Could you check a few things on this model? Use its own coordinates, in mm. A direction names the side the tool comes from. Give positions to 0.01 mm unless a question says otherwise; leave off trailing zeros. Loops run counter-clockwise (first coordinate to the right, second up) from the corner with the lowest first, then second, coordinate; pieces in that order, holes last. Notation, with made-up numbers: M -11.75,22 L 23.25,22 A34 ccw 23.25,55 Z; hole C -6,61.25 d11. An arc over 180 degrees is marked long. Use a Markdown table: item, result. Add a question column.
1) Suppose I cut it at B-B on x = 40.5. List the corners of the cut face in (y, z) for me.
2) Will these pins go through, and if not, where does the flat tip stop? pin 1 Ø4 at (x, z) = (105.5, 3.5) entering from -Y; pin 2 Ø5.5 at (x, y) = (18.2, 54.31) entering from +Z; pin 3 Ø2 at (x, z) = (191, 12.5) entering from +Y.
3) Suppose I cut it at A-A on y = 44. List the corners of the cut face in (x, z) for me, and give its area (3 significant figures).
4) We'd pull the mould along X, two halves only. Please class faces 1 (the cylindrical face through (20.89, 57.91, 12.29)), 2 (the cylindrical face through (-2.896, 24.969, 7.395)), 3 (the flat face through (217.772, 56.913, 7.395)): +X half, -X half, draft (parallel to the pull), parting line (faces both ways), or undercut.
5) If I drill on line 1 along Y through (x, z) = (75, 10.75); line 2 along X through (y, z) = (92.5, 13); line 3 along Y through (x, z) = (119, 9.5), over which ranges is the centre line in solid material (lowest first)? Write a range as [from, to].
6) Which directions (+Z, -Z, +X, -X, +Y, -Y) give clear straight access to the entire face, cutting with the end or side of a thin tool? Please do faces 4 (the cylindrical face through (229.443, 8.896, 7.395)), 5 (the cylindrical face through (172.725, 98.745, 7.395)), 6 (the flat face through (61, 88, 6.5)), 7 (the cylindrical face through (57.199, 98.723, 7.395)), 8 (the flat face through (169, 88, 8.5)).
```python
from build123d import *

# Parameters (mm, degrees)
EXTRUDE_7_DEPTH     = 15
CUT_EXTRUDE_1_DEPTH = 257.870857521
RIB_4_REACH         = 258.542
SKETCH_7_WALL_W     = 532.538559092
SKETCH_7_WALL_H     = 2
RIB_5_REACH         = 258.542
SKETCH_8_WALL_W     = 532.538559092
SKETCH_8_WALL_H     = 2
CUT_EXTRUDE_2_DEPTH = 257.870857521
CUT_EXTRUDE_3_DEPTH = 10
CUT_EXTRUDE_4_DEPTH = 257.870857521
EXTRUDE_8_DEPTH     = 2


with BuildPart() as part:
    # 草图3 → 凸台-拉伸7 (new body)
    with BuildSketch(Plane.XY):
        with BuildLine():
            Line((226.107883645, 4.564084021), (228.1313581, 6.587558476))
            ThreePointArc((228.1313581, 6.587558476), (229.452157682, 8.933123872), (229.365360937, 11.623598716))
            ThreePointArc((229.365360937, 11.623598716), (202.204022959, 54.721265071), (157.336152658, 78.846383531))
            ThreePointArc((157.336152658, 78.846383531), (156.176241581, 79.053674225), (155, 79.123092382))
            Line((155, 79.123092382), (75, 79.123092382))
            ThreePointArc((75, 79.123092382), (73.823758419, 79.053674225), (72.663847342, 78.846383531))
            ThreePointArc((72.663847342, 78.846383531), (27.795977041, 54.721265071), (0.634639063, 11.623598716))
            ThreePointArc((0.634639063, 11.623598716), (0.547842318, 8.933123872), (1.8686419, 6.587558476))
            Line((1.8686419, 6.587558476), (3.892116355, 4.564084021))
            ThreePointArc((3.892116355, 4.564084021), (4.038087075, 4.232340324), (3.921585186, 3.889136825))
            Line((3.921585186, 3.889136825), (3.278797577, 3.123092382))
            ThreePointArc((3.278797577, 3.123092382), (2.939119693, 2.946368462), (2.574022538, 3.0617655))
            ThreePointArc((2.574022538, 3.0617655), (-3.997102919, -0.152211219), (2.799416849, -2.857142857))
            ThreePointArc((2.799416849, -2.857142857), (4.567091757, -2.875182235), (4.549052379, -4.642857143))
            ThreePointArc((4.549052379, -4.642857143), (-2.777041025, -5.876907618), (-6.475265538, 0.566512328))
            Line((-6.475265538, 0.566512328), (-5.60370811, 10.528459309))
            ThreePointArc((-5.60370811, 10.528459309), (-2.837136411, 25.169145871), (2.769030559, 38.974018703))
            Line((2.769030559, 38.974018703), (21.426225279, 74.356346003))
            ThreePointArc((21.426225279, 74.356346003), (23.699524873, 77.563248735), (26.727922901, 80.069425417))
            Line((26.727922901, 80.069425417), (54.688883256, 97.596110672))
            ThreePointArc((54.688883256, 97.596110672), (57.236866172, 98.733768292), (60, 99.123092382))
            Line((60, 99.123092382), (170, 99.123092382))
            ThreePointArc((170, 99.123092382), (172.763133828, 98.733768292), (175.311116744, 97.596110672))
            Line((175.311116744, 97.596110672), (203.272077099, 80.069425417))
            ThreePointArc((203.272077099, 80.069425417), (206.300475127, 77.563248735), (208.573774721, 74.356346003))
            Line((208.573774721, 74.356346003), (227.230969441, 38.974018703))
            ThreePointArc((227.230969441, 38.974018703), (232.837136411, 25.169145871), (235.60370811, 10.528459309))
            Line((235.60370811, 10.528459309), (236.475265538, 0.566512328))
            ThreePointArc((236.475265538, 0.566512328), (232.777041025, -5.876907618), (225.450947621, -4.642857143))
            ThreePointArc((225.450947621, -4.642857143), (225.432908243, -2.875182235), (227.200583151, -2.857142857))
            ThreePointArc((227.200583151, -2.857142857), (233.997102919, -0.152211219), (227.425977462, 3.0617655))
            ThreePointArc((227.425977462, 3.0617655), (227.060880307, 2.946368462), (226.721202423, 3.123092382))
            Line((226.721202423, 3.123092382), (226.078414814, 3.889136825))
            ThreePointArc((226.078414814, 3.889136825), (225.961912925, 4.232340324), (226.107883645, 4.564084021))
        make_face()
        with BuildLine():
            Line((155, 79.123092382), (151.5, 79.123092382))
            ThreePointArc((151.5, 79.123092382), (151.75, 79.056105084), (151.933012702, 78.873092382))
            Line((151.933012702, 78.873092382), (153.208862747, 76.663255282))
            ThreePointArc((153.208862747, 76.663255282), (153.460925165, 76.447146931), (153.792778177, 76.436570515))
            ThreePointArc((153.792778177, 76.436570515), (158.62462258, 70.93131487), (151.301621364, 71.099282859))
            ThreePointArc((151.301621364, 71.099282859), (149.669687564, 71.778835706), (148.990134717, 70.146901906))
            ThreePointArc((148.990134717, 70.146901906), (155.784690615, 66.170630787), (161.428180194, 71.659505648))
            ThreePointArc((161.428180194, 71.659505648), (163.815160833, 75.214538736), (168.0781083, 75.6185384))
            ThreePointArc((168.0781083, 75.6185384), (162.752422297, 77.383187743), (157.336152658, 78.846383531))
            ThreePointArc((157.336152658, 78.846383531), (156.176241581, 79.053674225), (155, 79.123092382))
        make_face()
        with BuildLine():
            ThreePointArc((72.663847342, 78.846383531), (67.247577703, 77.383187743), (61.9218917, 75.6185384))
            ThreePointArc((61.9218917, 75.6185384), (66.184839167, 75.214538736), (68.571819806, 71.659505648))
            ThreePointArc((68.571819806, 71.659505648), (74.215309385, 66.170630787), (81.009865283, 70.146901906))
            ThreePointArc((81.009865283, 70.146901906), (80.330312436, 71.778835706), (78.698378636, 71.099282859))
            ThreePointArc((78.698378636, 71.099282859), (71.37537742, 70.93131487), (76.207221823, 76.436570515))
            ThreePointArc((76.207221823, 76.436570515), (76.539074835, 76.447146931), (76.791137253, 76.663255282))
            Line((76.791137253, 76.663255282), (78.066987298, 78.873092382))
            ThreePointArc((78.066987298, 78.873092382), (78.25, 79.056105084), (78.5, 79.123092382))
            Line((78.5, 79.123092382), (75, 79.123092382))
            ThreePointArc((75, 79.123092382), (73.823758419, 79.053674225), (72.663847342, 78.846383531))
        make_face()
    extrude(amount=EXTRUDE_7_DEPTH)

    # 草图6 → 切除-拉伸1 (cut, through all)
    with BuildSketch(Plane.XY.offset(15)):
        with BuildLine():
            ThreePointArc((58.67439973, 95.652604272), (57.292832816, 95.457942227), (56.018841358, 94.889113416))
            Line((56.018841358, 94.889113416), (51.236866172, 91.891642195))
            Line((51.236866172, 91.891642195), (51.236866172, 74.437432673))
            ThreePointArc((51.236866172, 74.437432673), (60.685741856, 78.429836873), (70.484678821, 81.463214092))
            ThreePointArc((70.484678821, 81.463214092), (71.026743583, 81.818757299), (71.236866172, 82.432022066))
            Line((71.236866172, 82.432022066), (71.236866172, 94.652604272))
            ThreePointArc((71.236866172, 94.652604272), (70.943972953, 95.359711053), (70.236866172, 95.652604272))
            Line((70.236866172, 95.652604272), (58.67439973, 95.652604272))
        make_face()
        with BuildLine():
            Line((51.236866172, 74.437432673), (51.236866172, 91.891642195))
            Line((51.236866172, 91.891642195), (25.036895933, 75.468793115))
            ThreePointArc((25.036895933, 75.468793115), (24.027429924, 74.633400887), (23.269663392, 73.56443331))
            Line((23.269663392, 73.56443331), (20.075243888, 67.506395211))
            ThreePointArc((20.075243888, 67.506395211), (21.629779543, 60.026321447), (29.268885543, 60.136521861))
            ThreePointArc((29.268885543, 60.136521861), (39.796372927, 67.988222639), (51.236866172, 74.437432673))
        make_face()
        with BuildLine():
            Line((178.763133828, 74.437432673), (178.763133828, 91.891642195))
            Line((178.763133828, 91.891642195), (173.981158642, 94.889113416))
            ThreePointArc((173.981158642, 94.889113416), (172.707167184, 95.457942227), (171.32560027, 95.652604272))
            Line((171.32560027, 95.652604272), (159.763133828, 95.652604272))
            ThreePointArc((159.763133828, 95.652604272), (159.056027047, 95.359711053), (158.763133828, 94.652604272))
            Line((158.763133828, 94.652604272), (158.763133828, 82.432022066))
            ThreePointArc((158.763133828, 82.432022066), (158.973256417, 81.818757299), (159.515321179, 81.463214092))
            ThreePointArc((159.515321179, 81.463214092), (169.314258144, 78.429836873), (178.763133828, 74.437432673))
        make_face()
        with BuildLine():
            Line((204.963104067, 75.468793115), (178.763133828, 91.891642195))
            Line((178.763133828, 91.891642195), (178.763133828, 74.437432673))
            ThreePointArc((178.763133828, 74.437432673), (190.203627073, 67.988222639), (200.731114457, 60.136521861))
            ThreePointArc((200.731114457, 60.136521861), (208.370220457, 60.026321447), (209.924756112, 67.506395211))
            Line((209.924756112, 67.506395211), (206.730336608, 73.56443331))
            ThreePointArc((206.730336608, 73.56443331), (205.972570076, 74.633400887), (204.963104067, 75.468793115))
        make_face()
    extrude(amount=-CUT_EXTRUDE_1_DEPTH, mode=Mode.SUBTRACT)

    # 草图7 wall → 筋4 (add, up to next)
    with BuildSketch(Plane(origin=(51.236866172, 83.164537434, 7.5), x_dir=(0, -1, 0), z_dir=(1, 0, 0)), mode=Mode.PRIVATE) as rib_4_sk1:
        Rectangle(SKETCH_7_WALL_W, SKETCH_7_WALL_H)
    rib_4_tool1 = extrude(rib_4_sk1.sketch, amount=RIB_4_REACH, mode=Mode.PRIVATE) - part.part
    add(rib_4_tool1.solids().sort_by_distance((51.236866172, 83.164537434, 7.5))[0])

    # 草图8 wall → 筋5 (add, up to next)
    with BuildSketch(Plane(origin=(178.763133828, 83.164537434, 7.5), x_dir=(0, -1, 0), z_dir=(1, 0, 0)), mode=Mode.PRIVATE) as rib_5_sk1:
        Rectangle(SKETCH_8_WALL_W, SKETCH_8_WALL_H)
    rib_5_tool1 = extrude(rib_5_sk1.sketch, amount=-RIB_5_REACH, mode=Mode.PRIVATE) - part.part
    add(rib_5_tool1.solids().sort_by_distance((178.763133828, 83.164537434, 7.5))[0])

    # 草图9 → 切除-拉伸2 (cut, through all)
    with BuildSketch(Plane.XY.offset(15)):
        with BuildLine():
            Line((76.236866172, 93.123092382), (153.763133828, 93.123092382))
            Line((153.763133828, 93.123092382), (153.763133828, 85.123092382))
            ThreePointArc((153.763133828, 85.123092382), (153.177347391, 83.70887882), (151.763133828, 83.123092382))
            Line((151.763133828, 83.123092382), (78.236866172, 83.123092382))
            ThreePointArc((78.236866172, 83.123092382), (76.822652609, 83.70887882), (76.236866172, 85.123092382))
            Line((76.236866172, 85.123092382), (76.236866172, 93.123092382))
        make_face()
    extrude(amount=-CUT_EXTRUDE_2_DEPTH, mode=Mode.SUBTRACT)

    # 草图10 → 切除-拉伸3 (cut)
    with BuildSketch(Plane(origin=(0, 99.123092382, 0), x_dir=(1, 0, 0), z_dir=(0, 1, 0))):
        with BuildLine():
            Line((152, -6.25), (78, -6.25))
            ThreePointArc((78, -6.25), (76.75, -7.5), (78, -8.75))
            Line((78, -8.75), (152, -8.75))
            ThreePointArc((152, -8.75), (153.25, -7.5), (152, -6.25))
        make_face()
    extrude(amount=-CUT_EXTRUDE_3_DEPTH, mode=Mode.SUBTRACT)

    # 草图11 → 切除-拉伸4 (cut, through all)
    with BuildSketch(Plane.XY.offset(15)):
        with BuildLine():
            Line((14.222124531, 56.406281397), (3.59559655, 36.253664848))
            ThreePointArc((3.59559655, 36.253664848), (4.660529559, 32.65450196), (8.285133372, 33.629336818))
            ThreePointArc((8.285133372, 33.629336818), (14.408945847, 42.791561817), (21.485479078, 51.239645835))
            ThreePointArc((21.485479078, 51.239645835), (20.80587389, 57.973042706), (14.222124531, 56.406281397))
        make_face()
        with BuildLine():
            Line((215.777875469, 56.406281397), (226.40440345, 36.253664848))
            ThreePointArc((226.40440345, 36.253664848), (225.339470441, 32.65450196), (221.714866628, 33.629336818))
            ThreePointArc((221.714866628, 33.629336818), (215.591054153, 42.791561817), (208.514520922, 51.239645835))
            ThreePointArc((208.514520922, 51.239645835), (209.19412611, 57.973042706), (215.777875469, 56.406281397))
        make_face()
    extrude(amount=-CUT_EXTRUDE_4_DEPTH, mode=Mode.SUBTRACT)

    # 草图12 → 凸台-拉伸8 (add, symmetric)
    with BuildSketch(Plane.XY.offset(7.5)):
        with BuildLine():
            Line((215.777875469, 56.406281397), (226.40440345, 36.253664848))
            ThreePointArc((226.40440345, 36.253664848), (225.339470441, 32.65450196), (221.714866628, 33.629336818))
            ThreePointArc((221.714866628, 33.629336818), (215.591054153, 42.791561817), (208.514520922, 51.239645835))
            ThreePointArc((208.514520922, 51.239645835), (209.19412611, 57.973042706), (215.777875469, 56.406281397))
        make_face()
        with BuildLine():
            Line((14.222124531, 56.406281397), (3.59559655, 36.253664848))
            ThreePointArc((3.59559655, 36.253664848), (4.660529559, 32.65450196), (8.285133372, 33.629336818))
            ThreePointArc((8.285133372, 33.629336818), (14.408945847, 42.791561817), (21.485479078, 51.239645835))
            ThreePointArc((21.485479078, 51.239645835), (20.80587389, 57.973042706), (14.222124531, 56.406281397))
        make_face()
    extrude(amount=EXTRUDE_8_DEPTH, both=True)


solid = part.part
```
Answer block:
| question | item | result |
|---|---|---|
| 1 | outline | M 64.78,0 L 68.44,0 L 68.44,15 L 64.78,15 Z; M 85.16,0 L 88.7,0 L 88.7,15 L 85.16,15 Z |
| 2 | pin 1 | stops at y = 79.12 |
| 2 | pin 2 | stops at z = 9.5 |
| 2 | pin 3 | stops at y = 88.39 |
| 3 | outline | M 5.42,0 L 7.68,0 L 7.68,5.5 L 15.33,5.5 L 15.33,0 L 17.87,0 L 17.87,15 L 15.33,15 L 15.33,9.5 L 7.68,9.5 L 7.68,15 L 5.42,15 Z; M 212.13,0 L 214.67,0 L 214.67,5.5 L 222.32,5.5 L 222.32,0 L 224.58,0 L 224.58,15 L 222.32,15 L 222.32,9.5 L 214.67,9.5 L 214.67,15 L 212.13,15 Z |
| 3 | area | 205 mm^2 |
| 4 | face 1 | undercut |
| 4 | face 2 | -X half |
| 4 | face 3 | +X half |
| 5 | line 1 | y = [66.12, 68.62], [76.62, 99.12] |
| 5 | line 2 | x = [46.56, 52.21], [71.24, 76.24], [153.76, 158.76], [177.79, 183.44] |
| 5 | line 3 | y = [79.12, 83.12], [93.12, 99.12] |
| 6 | face 4 | +Z, -Z |
| 6 | face 5 | +Z, -Z, +X, +Y |
| 6 | face 6 | -Z |
| 6 | face 7 | +Z, -Z, -X, +Y |
| 6 | face 8 | +Z |
